```python
from build123d import *

# Parameters (mm, degrees)
SKETCH_R      = 1.5
PAD_DEPTH     = 2
SKETCH001_R   = 1.1
SKETCH001_R_2 = 1.6
POCKET_DEPTH  = 2.001


with BuildPart() as part:
    # Sketch → Pad (new body)
    with BuildSketch(Plane.XY):
        with BuildLine():
            Line((0, 68), (0, 12))
            ThreePointArc((12, 0), (8.485281, 8.485281), (0, 12))
            Line((12, 0), (137, 0))
            ThreePointArc((149, 12), (140.514719, 8.485281), (137, 0))
            Line((149, 12), (149, 68))
            ThreePointArc((137, 80), (140.514719, 71.514719), (149, 68))
            Line((137, 80), (12, 80))
            ThreePointArc((0, 68), (8.485281, 71.514719), (12, 80))
        make_face()
        with Locations((16, 73.5)):
            Circle(SKETCH_R, mode=Mode.SUBTRACT)
        with Locations((7.5, 40)):
            Circle(SKETCH_R, mode=Mode.SUBTRACT)
        with Locations((16, 6.5)):
            Circle(SKETCH_R, mode=Mode.SUBTRACT)
        with Locations((133, 6.5)):
            Circle(SKETCH_R, mode=Mode.SUBTRACT)
        with Locations((141.5, 40)):
            Circle(SKETCH_R, mode=Mode.SUBTRACT)
        with Locations((133, 73.5)):
            Circle(SKETCH_R, mode=Mode.SUBTRACT)
    extrude(amount=PAD_DEPTH)

    # Sketch001 (on Face16 of Pad) → Pocket (cut, through all)
    with BuildSketch(Plane.XY.offset(2)):
        with Locations((6, 66)):
            Circle(SKETCH001_R)
        with Locations((30, 66)):
            Circle(SKETCH001_R)
        with Locations((30, 16)):
            Circle(SKETCH001_R)
        with Locations((6, 16)):
            Circle(SKETCH001_R)
        with Locations((45, 22)):
            Circle(SKETCH001_R_2)
        with Locations((70, 22)):
            Circle(SKETCH001_R_2)
        with Locations((70, 76)):
            Circle(SKETCH001_R_2)
        with Locations((45, 76)):
            Circle(SKETCH001_R_2)
        with Locations((85, 76)):
            Circle(SKETCH001_R_2)
        with Locations((85, 52)):
            Circle(SKETCH001_R_2)
        with Locations((121, 52)):
            Circle(SKETCH001_R_2)
        with Locations((121, 76)):
            Circle(SKETCH001_R_2)
    extrude(amount=-POCKET_DEPTH, mode=Mode.SUBTRACT)


solid = part.part
```
Design review of the part built by this model. Coordinates are the model's own, in mm. Coordinates: 2 decimals unless noted, no trailing zeros. Loops run counter-clockwise (first coordinate to the right, second up) from the corner with the lowest first, then second, coordinate; pieces in that order, holes last.
Q1. For pin 1 (1.5 mm diameter, centred on x = 118, y = 56, fed in from -Z); pin 2 (2.5 mm diameter, centred on x = 121, y = 76, fed in from -Z), all flat-tipped, find the tip position at first contact; note any pin that passes through.
Reported:
pin 1: stops at z = 0
pin 2: passes through
Q2. We need section C-C on z = 1.3. State how many separate pieces and enclosed holes the cut face has, and give its area (3 significant figures).
Reported:
separate pieces: 1
enclosed holes: 18
area: 11,300 mm2
Q3. We need section A-A on x = 121. State the section outline as (y, z) points.
Reported:
outline: (0, 0) - (50.4, 0) - (50.4, 2) - (0, 2) - close; (53.6, 0) - (74.4, 0) - (74.4, 2) - (53.6, 2) - close; (77.6, 0) - (80, 0) - (80, 2) - (77.6, 2) - close
Q4. We need section B-B on y = 22. State the section outline as (x, z) points.
Reported:
outline: (0, 0) - (43.4, 0) - (43.4, 2) - (0, 2) - close; (46.6, 0) - (68.4, 0) - (68.4, 2) - (46.6, 2) - close; (71.6, 0) - (149, 0) - (149, 2) - (71.6, 2) - close
Q5. The part is to be moulded in two halves that separate along X. For faces 1 (the face through (8.39, 71.42, 0.99)), 2 (the face through (73, 41, 2)), 3 (the face through (44.792, 77.586, 1.014)), 4 (the face through (83.4, 76.07, 1.01)), say which applies: +X half, -X half, draft (parallel to the pull), parting line (faces both ways), or undercut.
Reported:
face 1: -X half
face 2: draft
face 3: undercut
face 4: undercut
Q6. To check wall thickness, follow line 1 (Y direction, x = 85, z = 0.65); line 2 (Y direction, x = 30, z = 1.15); line 3 (X direction, y = 66, z = 0.7). State the ranges of each line that lie inside material, in increasing order.
Reported:
line 1: y = 0 to 50.4, 53.6 to 74.4, 77.6 to 80
line 2: y = 0 to 14.9, 17.1 to 64.9, 67.1 to 80
line 3: x = 0 to 4.9, 7.1 to 28.9, 31.1 to 149
